from build123d import *

# Parameters (mm, degrees)
IZIM1_W                     = 100
IZIM1_H                     = 100
IZIM1_R                     = 0.75
Y_KSEKLIK_EKSTR_ZYON1_DEPTH = 3
IZIM2_R                     = 6
KES_EKSTR_ZYON1_DEPTH       = 4
KES_EKSTR_ZYON2_DEPTH       = 4
KES_EKSTR_ZYON3_DEPTH       = 4


with BuildPart() as part:
    # Çizim1 → Yükseklik-Ekstrüzyon1 (new body)
    with BuildSketch(Plane(origin=(0, 0, 0), x_dir=(1, 0, 0), z_dir=(0, 1, 0))):
        Rectangle(IZIM1_W, IZIM1_H)
        with Locations(Location((-35, 35, 0), (0, 0, 270))):
            Circle(IZIM1_R, mode=Mode.SUBTRACT)
        with Locations(Location((35, 35, 0), (0, 0, 270))):
            Circle(IZIM1_R, mode=Mode.SUBTRACT)
        with Locations(Location((35, -35, 0), (0, 0, 270))):
            Circle(IZIM1_R, mode=Mode.SUBTRACT)
        with Locations(Location((-35, -35, 0), (0, 0, 270))):
            Circle(IZIM1_R, mode=Mode.SUBTRACT)
    extrude(amount=-Y_KSEKLIK_EKSTR_ZYON1_DEPTH)

    # Çizim2 → Kes-Ekstrüzyon1 (cut)
    with BuildSketch(Plane(origin=(0, 0, 0), x_dir=(1, 0, 0), z_dir=(0, 1, 0))):
        with Locations(Location((0, 0, 0), (0, 0, 270))):
            Circle(IZIM2_R)
    extrude(amount=-KES_EKSTR_ZYON1_DEPTH, mode=Mode.SUBTRACT)

    # Çizim3 → Kes-Ekstrüzyon2 (cut)
    with BuildSketch(Plane(origin=(0, 0, 0), x_dir=(1, 0, 0), z_dir=(0, 1, 0))):
        with BuildLine():
            Line((-50, 30.263704164), (-50, 50))
            Line((-50, 50), (-30.263704164, 50))
            ThreePointArc((-30.263704164, 50), (-44.219372785, 44.219372785), (-50, 30.263704164))
        make_face()
        with BuildLine():
            Line((50, 50), (50, 30.263704164))
            ThreePointArc((50, 30.263704164), (44.219372785, 44.219372785), (30.263704164, 50))
            Line((30.263704164, 50), (50, 50))
        make_face()
        with BuildLine():
            Line((50, -50), (30.263704164, -50))
            ThreePointArc((30.263704164, -50), (44.219372785, -44.219372785), (50, -30.263704164))
            Line((50, -30.263704164), (50, -50))
        make_face()
        with BuildLine():
            Line((-50, -50), (-50, -30.263704164))
            ThreePointArc((-50, -30.263704164), (-44.219372785, -44.219372785), (-30.263704164, -50))
            Line((-30.263704164, -50), (-50, -50))
        make_face()
    extrude(amount=-KES_EKSTR_ZYON2_DEPTH, mode=Mode.SUBTRACT)

    # Çizim4 → Kes-Ekstrüzyon3 (cut)
    with BuildSketch(Plane(origin=(0, 0, 0), x_dir=(1, 0, 0), z_dir=(0, 1, 0))):
        with BuildLine():
            Line((-9.174701876, -5.841446321), (-9.174701876, 5.841446321))
            ThreePointArc((-9.174701876, 5.841446321), (-10.674701876, 7.341446321), (-12.174701876, 5.841446321))
            Line((-12.174701876, 5.841446321), (-12.174701876, -5.841446321))
            ThreePointArc((-12.174701876, -5.841446321), (-10.674701876, -7.341446321), (-9.174701876, -5.841446321))
        make_face()
        with BuildLine():
            Line((-17.174701876, -5.841446321), (-17.174701876, 5.841446321))
            ThreePointArc((-17.174701876, 5.841446321), (-18.674701876, 7.341446321), (-20.174701876, 5.841446321))
            Line((-20.174701876, 5.841446321), (-20.174701876, -5.841446321))
            ThreePointArc((-20.174701876, -5.841446321), (-18.674701876, -7.341446321), (-17.174701876, -5.841446321))
        make_face()
        with BuildLine():
            Line((-25.174701876, -5.841446321), (-25.174701876, 5.841446321))
            ThreePointArc((-25.174701876, 5.841446321), (-26.674701876, 7.341446321), (-28.174701876, 5.841446321))
            Line((-28.174701876, 5.841446321), (-28.174701876, -5.841446321))
            ThreePointArc((-28.174701876, -5.841446321), (-26.674701876, -7.341446321), (-25.174701876, -5.841446321))
        make_face()
        with BuildLine():
            Line((-33.174701876, -5.841446321), (-33.174701876, 5.841446321))
            ThreePointArc((-33.174701876, 5.841446321), (-34.674701876, 7.341446321), (-36.174701876, 5.841446321))
            Line((-36.174701876, 5.841446321), (-36.174701876, -5.841446321))
            ThreePointArc((-36.174701876, -5.841446321), (-34.674701876, -7.341446321), (-33.174701876, -5.841446321))
        make_face()
        with BuildLine():
            Line((-41.174701876, -5.841446321), (-41.174701876, 5.841446321))
            ThreePointArc((-41.174701876, 5.841446321), (-42.674701876, 7.341446321), (-44.174701876, 5.841446321))
            Line((-44.174701876, 5.841446321), (-44.174701876, -5.841446321))
            ThreePointArc((-44.174701876, -5.841446321), (-42.674701876, -7.341446321), (-41.174701876, -5.841446321))
        make_face()
        with BuildLine():
            Line((-5.841446321, 9.174701876), (5.841446321, 9.174701876))
            ThreePointArc((5.841446321, 9.174701876), (7.341446321, 10.674701876), (5.841446321, 12.174701876))
            Line((5.841446321, 12.174701876), (-5.841446321, 12.174701876))
            ThreePointArc((-5.841446321, 12.174701876), (-7.341446321, 10.674701876), (-5.841446321, 9.174701876))
        make_face()
        with BuildLine():
            Line((-5.841446321, 17.174701876), (5.841446321, 17.174701876))
            ThreePointArc((5.841446321, 17.174701876), (7.341446321, 18.674701876), (5.841446321, 20.174701876))
            Line((5.841446321, 20.174701876), (-5.841446321, 20.174701876))
            ThreePointArc((-5.841446321, 20.174701876), (-7.341446321, 18.674701876), (-5.841446321, 17.174701876))
        make_face()
        with BuildLine():
            Line((-5.841446321, 25.174701876), (5.841446321, 25.174701876))
            ThreePointArc((5.841446321, 25.174701876), (7.341446321, 26.674701876), (5.841446321, 28.174701876))
            Line((5.841446321, 28.174701876), (-5.841446321, 28.174701876))
            ThreePointArc((-5.841446321, 28.174701876), (-7.341446321, 26.674701876), (-5.841446321, 25.174701876))
        make_face()
        with BuildLine():
            Line((-5.841446321, 33.174701876), (5.841446321, 33.174701876))
            ThreePointArc((5.841446321, 33.174701876), (7.341446321, 34.674701876), (5.841446321, 36.174701876))
            Line((5.841446321, 36.174701876), (-5.841446321, 36.174701876))
            ThreePointArc((-5.841446321, 36.174701876), (-7.341446321, 34.674701876), (-5.841446321, 33.174701876))
        make_face()
        with BuildLine():
            Line((-5.841446321, 41.174701876), (5.841446321, 41.174701876))
            ThreePointArc((5.841446321, 41.174701876), (7.341446321, 42.674701876), (5.841446321, 44.174701876))
            Line((5.841446321, 44.174701876), (-5.841446321, 44.174701876))
            ThreePointArc((-5.841446321, 44.174701876), (-7.341446321, 42.674701876), (-5.841446321, 41.174701876))
        make_face()
        with BuildLine():
            Line((9.174701876, 5.841446321), (9.174701876, -5.841446321))
            ThreePointArc((9.174701876, -5.841446321), (10.674701876, -7.341446321), (12.174701876, -5.841446321))
            Line((12.174701876, -5.841446321), (12.174701876, 5.841446321))
            ThreePointArc((12.174701876, 5.841446321), (10.674701876, 7.341446321), (9.174701876, 5.841446321))
        make_face()
        with BuildLine():
            Line((17.174701876, 5.841446321), (17.174701876, -5.841446321))
            ThreePointArc((17.174701876, -5.841446321), (18.674701876, -7.341446321), (20.174701876, -5.841446321))
            Line((20.174701876, -5.841446321), (20.174701876, 5.841446321))
            ThreePointArc((20.174701876, 5.841446321), (18.674701876, 7.341446321), (17.174701876, 5.841446321))
        make_face()
        with BuildLine():
            Line((25.174701876, 5.841446321), (25.174701876, -5.841446321))
            ThreePointArc((25.174701876, -5.841446321), (26.674701876, -7.341446321), (28.174701876, -5.841446321))
            Line((28.174701876, -5.841446321), (28.174701876, 5.841446321))
            ThreePointArc((28.174701876, 5.841446321), (26.674701876, 7.341446321), (25.174701876, 5.841446321))
        make_face()
        with BuildLine():
            Line((33.174701876, 5.841446321), (33.174701876, -5.841446321))
            ThreePointArc((33.174701876, -5.841446321), (34.674701876, -7.341446321), (36.174701876, -5.841446321))
            Line((36.174701876, -5.841446321), (36.174701876, 5.841446321))
            ThreePointArc((36.174701876, 5.841446321), (34.674701876, 7.341446321), (33.174701876, 5.841446321))
        make_face()
        with BuildLine():
            Line((41.174701876, 5.841446321), (41.174701876, -5.841446321))
            ThreePointArc((41.174701876, -5.841446321), (42.674701876, -7.341446321), (44.174701876, -5.841446321))
            Line((44.174701876, -5.841446321), (44.174701876, 5.841446321))
            ThreePointArc((44.174701876, 5.841446321), (42.674701876, 7.341446321), (41.174701876, 5.841446321))
        make_face()
        with BuildLine():
            Line((5.841446321, -9.174701876), (-5.841446321, -9.174701876))
            ThreePointArc((-5.841446321, -9.174701876), (-7.341446321, -10.674701876), (-5.841446321, -12.174701876))
            Line((-5.841446321, -12.174701876), (5.841446321, -12.174701876))
            ThreePointArc((5.841446321, -12.174701876), (7.341446321, -10.674701876), (5.841446321, -9.174701876))
        make_face()
        with BuildLine():
            Line((5.841446321, -17.174701876), (-5.841446321, -17.174701876))
            ThreePointArc((-5.841446321, -17.174701876), (-7.341446321, -18.674701876), (-5.841446321, -20.174701876))
            Line((-5.841446321, -20.174701876), (5.841446321, -20.174701876))
            ThreePointArc((5.841446321, -20.174701876), (7.341446321, -18.674701876), (5.841446321, -17.174701876))
        make_face()
        with BuildLine():
            Line((5.841446321, -25.174701876), (-5.841446321, -25.174701876))
            ThreePointArc((-5.841446321, -25.174701876), (-7.341446321, -26.674701876), (-5.841446321, -28.174701876))
            Line((-5.841446321, -28.174701876), (5.841446321, -28.174701876))
            ThreePointArc((5.841446321, -28.174701876), (7.341446321, -26.674701876), (5.841446321, -25.174701876))
        make_face()
        with BuildLine():
            Line((5.841446321, -33.174701876), (-5.841446321, -33.174701876))
            ThreePointArc((-5.841446321, -33.174701876), (-7.341446321, -34.674701876), (-5.841446321, -36.174701876))
            Line((-5.841446321, -36.174701876), (5.841446321, -36.174701876))
            ThreePointArc((5.841446321, -36.174701876), (7.341446321, -34.674701876), (5.841446321, -33.174701876))
        make_face()
        with BuildLine():
            Line((5.841446321, -41.174701876), (-5.841446321, -41.174701876))
            ThreePointArc((-5.841446321, -41.174701876), (-7.341446321, -42.674701876), (-5.841446321, -44.174701876))
            Line((-5.841446321, -44.174701876), (5.841446321, -44.174701876))
            ThreePointArc((5.841446321, -44.174701876), (7.341446321, -42.674701876), (5.841446321, -41.174701876))
        make_face()
        with BuildLine():
            ThreePointArc((-12.174701876, 32.099731448), (-9.599731448, 34.674701876), (-12.174701876, 37.249672305))
            ThreePointArc((-12.174701876, 37.249672305), (-29.905383504, 29.905383504), (-37.249672305, 12.174701876))
            ThreePointArc((-37.249672305, 12.174701876), (-34.674701876, 9.599731448), (-32.099731448, 12.174701876))
            ThreePointArc((-32.099731448, 12.174701876), (-26.263825402, 26.263825402), (-12.174701876, 32.099731448))
        make_face()
        with BuildLine():
            ThreePointArc((32.099731448, 12.174701876), (34.674701876, 9.599731448), (37.249672305, 12.174701876))
            ThreePointArc((37.249672305, 12.174701876), (29.905383504, 29.905383504), (12.174701876, 37.249672305))
            ThreePointArc((12.174701876, 37.249672305), (9.599731448, 34.674701876), (12.174701876, 32.099731448))
            ThreePointArc((12.174701876, 32.099731448), (26.263825402, 26.263825402), (32.099731448, 12.174701876))
        make_face()
        with BuildLine():
            ThreePointArc((12.174701876, -32.099731448), (9.599731448, -34.674701876), (12.174701876, -37.249672305))
            ThreePointArc((12.174701876, -37.249672305), (29.905383504, -29.905383504), (37.249672305, -12.174701876))
            ThreePointArc((37.249672305, -12.174701876), (34.674701876, -9.599731448), (32.099731448, -12.174701876))
            ThreePointArc((32.099731448, -12.174701876), (26.263825402, -26.263825402), (12.174701876, -32.099731448))
        make_face()
        with BuildLine():
            ThreePointArc((-32.099731448, -12.174701876), (-34.674701876, -9.599731448), (-37.249672305, -12.174701876))
            ThreePointArc((-37.249672305, -12.174701876), (-29.905383504, -29.905383504), (-12.174701876, -37.249672305))
            ThreePointArc((-12.174701876, -37.249672305), (-9.599731448, -34.674701876), (-12.174701876, -32.099731448))
            ThreePointArc((-12.174701876, -32.099731448), (-26.263825402, -26.263825402), (-32.099731448, -12.174701876))
        make_face()
    extrude(amount=-KES_EKSTR_ZYON3_DEPTH, mode=Mode.SUBTRACT)


solid = part.part
Build history of the part. All positions in model axes, mm. Round coordinates to 2 decimals unless told otherwise and drop trailing zeros. Write each loop counter-clockwise with the first axis right and the second up, starting at its lowest first coordinate (ties: lowest second). Pieces come first, ordered by that corner, then holes. Notation, with made-up numbers: M 62.25,68 L 99.25,68 A27 cw 99.25,102 Z; hole C 59,52.25 d4. An arc over 180 degrees is marked long. Answer in a Markdown table with one row per item.
1. Probe L1, parallel to Z at x = -35, y = -1.2; L2, parallel to X at y = -0.75, z = -34.5. List the from-to ranges inside material, lowest first. Write a range as [from, to].
Geometry check:
| item | result |
|---|---|
| L1 | [-49.42, -35.75], [-34.25, -22.56], [-9.62, -7.31], [7.31, 9.62], [22.56, 34.25], [35.75, 49.42] |
| L2 | [-49.54, -35.56], [-34.44, -23.59], [-9.61, -7.33], [7.33, 9.61], [23.59, 34.44], [35.56, 49.54] |
2. Saw through at B-B (z = -22). List the corners of the cut face in (x, y), and give its area (3 significant figures).
Geometry check:
| item | result |
|---|---|
| outline | M -50,-3 L -35.24,-3 L -35.24,0 L -50,0 Z; M -29.51,-3 L 29.51,-3 L 29.51,0 L -29.51,0 Z; M 35.24,-3 L 50,-3 L 50,0 L 35.24,0 Z |
| area | 266 mm2 |
3. Saw through at C-C (x = 0). State how many separate pieces and enclosed holes the cut face has, and give its area (3 significant figures).
Geometry check:
| item | result |
|---|---|
| separate pieces | 12 |
| enclosed holes | 0 |
| area | 174 mm2 |
4. Saw through at A-A (x = 13.5). List the corners of the cut face in (y, z).
Geometry check:
| item | result |
|---|---|
| outline | M -3,-50 L 0,-50 L 0,-37.21 L -3,-37.21 Z; M -3,-32.06 L 0,-32.06 L 0,32.06 L -3,32.06 Z; M -3,37.21 L 0,37.21 L 0,50 L -3,50 Z |
5. Mould opens along X. For faces 1 (the face through (26.64, -1.48, 7.34)), 2 (the face through (-44.065, -1.479, -44.372)) say: +X half, -X half, draft (parallel to the pull), parting line (faces both ways), or undercut.
Geometry check:
| item | result |
|---|---|
| face 1 | undercut |
| face 2 | -X half |
6. Flat gauge pin, fed straight in: P1, Ø1, axis at y = -0.5, z = -36, coming from the +X side. Where does the tip first touch, or does it go through?
Geometry check:
| item | result |
|---|---|
| P1 | x = 49.29 |
